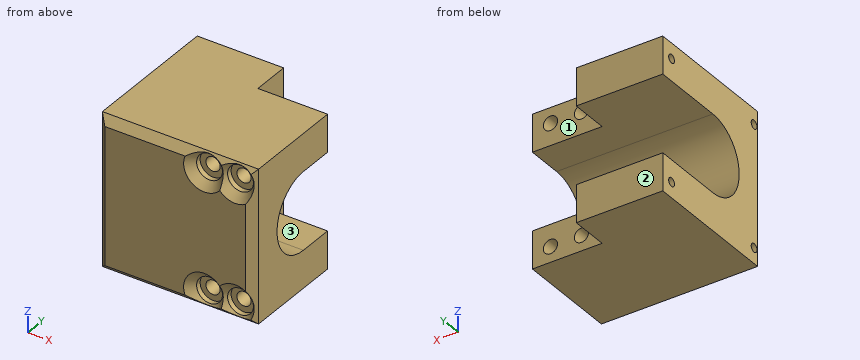
from build123d import *

# Parameters (mm, degrees)
BOSS_EXTRUDE1_DEPTH            = 59
SKETCH2_R                      = 1.65
CUT_EXTRUDE1_DEPTH             = 30
CBORE_FOR_M5_SHCS1_D           = 5.5
CBORE_FOR_M5_SHCS1_DEPTH       = 98.347633298
CBORE_FOR_M5_SHCS1_CBORE_D     = 10
CBORE_FOR_M5_SHCS1_CBORE_DEPTH = 5
CBORE_FOR_M5_SHCS1_TIP         = 1.652366702
CUT_EXTRUDE2_DEPTH             = 107.612616514
CHAMFER1_SIZE                  = 3


with BuildPart() as part:
    # Sketch1 → Boss-Extrude1 (new body)
    with BuildSketch(Plane.XY):
        Polygon((60.5, 22.7), (60.5, 50.3), (58.5, 50.3), (33.5, 50.3), (33.5, 65), (10, 65), (0, 65), (0, 8), (10, 8), (33.5, 8), (60.5, 8), align=None)
    extrude(amount=-BOSS_EXTRUDE1_DEPTH)

    # Sketch2 → Cut-Extrude1 (cut)
    with BuildSketch(Plane.ZY):
        with Locations((-6, 13)):
            Circle(SKETCH2_R)
        with Locations((-6, 60)):
            Circle(SKETCH2_R)
        with Locations((-53, 13)):
            Circle(SKETCH2_R)
        with Locations((-53, 60)):
            Circle(SKETCH2_R)
    extrude(amount=-CUT_EXTRUDE1_DEPTH, mode=Mode.SUBTRACT)

    # CBORE for M5 SHCS1
    with Locations(Plane(origin=(0, 8, 0), x_dir=(-1, 0, 0), z_dir=(0, -1, 0))):
        with Locations((-53.5, 6), (-41.5, 6), (-41.5, 53), (-53.5, 53)):
            CounterBoreHole(CBORE_FOR_M5_SHCS1_D / 2, CBORE_FOR_M5_SHCS1_CBORE_D / 2, CBORE_FOR_M5_SHCS1_CBORE_DEPTH, depth=CBORE_FOR_M5_SHCS1_DEPTH)
            with Locations((0, 0, -(CBORE_FOR_M5_SHCS1_DEPTH + CBORE_FOR_M5_SHCS1_TIP / 2))):  # 118° drill point
                Cone(0, CBORE_FOR_M5_SHCS1_D / 2, CBORE_FOR_M5_SHCS1_TIP, mode=Mode.SUBTRACT)

    # Sketch7 → Cut-Extrude2 (cut, through all)
    with BuildSketch(Plane.ZY):
        with BuildLine():
            Line((-14.5, 36.5), (-14.5, 65))
            Line((-14.5, 65), (-44.5, 65))
            Line((-44.5, 65), (-44.5, 36.5))
            ThreePointArc((-44.5, 36.5), (-29.5, 21.5), (-14.5, 36.5))
        make_face()
    extrude(amount=-CUT_EXTRUDE2_DEPTH, mode=Mode.SUBTRACT)

    # Chamfer1
    # the kernel refuses this chamfer: 3 mm, written as the material it takes off along each edge
    with BuildSketch(Plane(origin=(68.215048964, 8, 0), x_dir=(0, -0.02749587661058649, -0.9996219169112968), z_dir=(-1, 0, 0))) as chamfer1_piece_1:
        Polygon((CHAMFER1_SIZE * 0.999621916911, -CHAMFER1_SIZE * 0.0274958766106), (-CHAMFER1_SIZE * 0.0274958766106, -CHAMFER1_SIZE * 0.999621916911), (0, 0), align=None)
    extrude(amount=75.930097928, mode=Mode.SUBTRACT)
    with BuildSketch(Plane(origin=(60.5, 8, 7.715048964), x_dir=(0.02749587661058678, 0.9996219169112968, 0), z_dir=(0, 0, -1)), Plane(origin=(0, 8, 7.715048964), x_dir=(0.9996219169112968, -0.02749587661058649, 0), z_dir=(0, 0, -1))) as chamfer1_piece_2:
        Polygon((CHAMFER1_SIZE * 0.999621916911, -CHAMFER1_SIZE * 0.0274958766106), (-CHAMFER1_SIZE * 0.0274958766106, -CHAMFER1_SIZE * 0.999621916911), (0, 0), align=None)
    extrude(amount=74.430097928, mode=Mode.SUBTRACT)
    with BuildSketch(Plane(origin=(-7.715048964, 8, -59), x_dir=(0, 0.9996219169112968, -0.02749587661058678), z_dir=(1, 0, 0))) as chamfer1_piece_3:
        Polygon((CHAMFER1_SIZE * 0.999621916911, CHAMFER1_SIZE * 0.0274958766106), (-CHAMFER1_SIZE * 0.0274958766106, CHAMFER1_SIZE * 0.999621916911), (0, 0), align=None)
    extrude(amount=75.930097928, mode=Mode.SUBTRACT)
    with BuildSketch(Plane(origin=(53.5, 8, -53), x_dir=(-1, 0, 0), z_dir=(0, 0, 1))) as chamfer1_piece_4:
        Polygon((5 + CHAMFER1_SIZE, 0), (5, -CHAMFER1_SIZE), (5, 0), align=None)
    revolve(axis=Axis((53.5, 8, -53), (0, -1, 0)), mode=Mode.SUBTRACT)
    with BuildSketch(Plane(origin=(41.5, 8, -53), x_dir=(-1, 0, 0), z_dir=(0, 0, 1))) as chamfer1_piece_5:
        Polygon((5 + CHAMFER1_SIZE, 0), (5, -CHAMFER1_SIZE), (5, 0), align=None)
    revolve(axis=Axis((41.5, 8, -53), (0, -1, 0)), mode=Mode.SUBTRACT)
    with BuildSketch(Plane(origin=(41.5, 8, -6), x_dir=(-1, 0, 0), z_dir=(0, 0, 1))) as chamfer1_piece_6:
        Polygon((5 + CHAMFER1_SIZE, 0), (5, -CHAMFER1_SIZE), (5, 0), align=None)
    revolve(axis=Axis((41.5, 8, -6), (0, -1, 0)), mode=Mode.SUBTRACT)
    with BuildSketch(Plane(origin=(53.5, 8, -6), x_dir=(-1, 0, 0), z_dir=(0, 0, 1))) as chamfer1_piece_7:
        Polygon((5 + CHAMFER1_SIZE, 0), (5, -CHAMFER1_SIZE), (5, 0), align=None)
    revolve(axis=Axis((53.5, 8, -6), (0, -1, 0)), mode=Mode.SUBTRACT)


solid = part.part
The listing builds one solid part. Answer for the finished solid, in the listing's coordinates (mm). Face numbers are marked on the shaded views. A direction names the side the tool comes from. Give positions to 0.01 mm unless a question says otherwise; leave off trailing zeros. Loops run counter-clockwise (first coordinate to the right, second up) from the corner with the lowest first, then second, coordinate; pieces in that order, holes last.
Item 1: A cutting plane is placed at B-B (x = 53.5). Give the vertices of the cut face in (y, z), then the cut area to 3 significant figures.
Derived:
outline: (8, -45) - (11, -48) - (13, -48) - (13, -50.25) - (50.3, -50.25) - (50.3, -44.5) - (36.5, -44.5) arc R15 cw to (36.5, -14.5) - (50.3, -14.5) - (50.3, -8.75) - (13, -8.75) - (13, -11) - (11, -11) - (8, -14) - close; (10.5, -58.5) - (11, -59) - (50.3, -59) - (50.3, -55.75) - (13, -55.75) - (13, -58) - (11, -58) - close; (10.5, -0.5) - (11, -1) - (13, -1) - (13, -3.25) - (50.3, -3.25) - (50.3, 0) - (11, 0) - close
area: 1,200 mm2
Item 2: A cutting plane is placed at C-C (x = 24.5). Give the vertices of the cut face in (y, z), then the cut area to 3 significant figures.
Derived:
outline: (8, -56) - (11, -59) - (65, -59) - (65, -44.5) - (36.5, -44.5) arc R15 cw to (36.5, -14.5) - (65, -14.5) - (65, 0) - (11, 0) - (8, -3) - close; hole circle Ø3.3 at (13, -53); hole circle Ø3.3 at (13, -6); hole circle Ø3.3 at (60, -53); hole circle Ø3.3 at (60, -6)
area: 2,110 mm2
Item 3: Each of these flat-tipped pins is pushed along its axis until it touches: pin 1 Ø12 at (x, y) = (54, 57) entering from -Z; pin 2 Ø3 at (x, z) = (51.5, -54.5) entering from -Y; pin 3 Ø9 at (x, z) = (41.5, -6) entering from +Y; pin 4 Ø11 at (x, z) = (43.5, -4.5) entering from -Y. Where does it stop, or does it pass through?
Derived:
pin 1: passes through
pin 2: stops at y = 13
pin 3: stops at y = 50.3
pin 4: stops at y = 8.86
Item 4: A cutting plane is placed at A-A (y = 60). Give the vertices of the cut face in (x, z), then the cut area to 4 significant figures.
Derived:
outline: (0, -59) - (33.5, -59) - (33.5, -44.5) - (0, -44.5) - (0, -51.35) - (30, -51.35) - (30, -54.65) - (0, -54.65) - close; (0, -14.5) - (33.5, -14.5) - (33.5, 0) - (0, 0) - (0, -4.35) - (30, -4.35) - (30, -7.65) - (0, -7.65) - close
area: 773.5 mm2
Item 5: Find the intervals of material crossed by line 1 along Y through (x, z) = (21.25, -53); line 2 along Z through (x, y) = (53.5, 12.5); line 3 along X through (y, z) = (12.2, -6), in increasing order.
Derived:
line 1: y = 8 to 11.35, 14.65 to 58.35, 61.65 to 65
line 2: z = -59 to -58, -48 to -11, -1 to 0
line 3: x = 30 to 36.5, 46.5 to 48.5, 58.5 to 60.5
Item 6: A tool of negligible diameter and unlimited length cuts with its end or side. For the marked faces 1, 2 and 3, from which of +Z, -Z, +X, -X, +Y, -Y can it reach the whole face along a straight path? Write none if from no direction.
Derived:
face 1: +Z, -Z, +X, +Y
face 2: +Z, -Z, +X, -X, +Y
face 3: +X, -X, +Y
Item 7: A cutting plane is placed at D-D (z = -29.5). Give the vertices of the cut face in (x, y).
Derived:
outline: (0, 11) - (3, 8) - (57.5, 8) - (60.5, 11) - (60.5, 21.5) - (0, 21.5) - close
